```python
from build123d import *

# Parameters (mm, degrees)
SKETCH2_R          = 1.93
CUT_EXTRUDE1_DEPTH = 19.1
CIRPATTERN1_COUNT  = 16
SKETCH3_W          = 1.65
SKETCH3_H          = 14.001
CIRPATTERN2_COUNT  = 2
CIRPATTERN2_ANGLE  = 90


with BuildPart() as part:
    # Sketch1 → Revolve1 (revolve)
    with BuildSketch(Plane.XY):
        Polygon((-11.25, 6.35), (16.75, 6.35), (16.75, 14), (9.55, 14), (9.55, 11.66), (-9.55, 11.66), (-9.55, 10), (-11.25, 10), align=None)
    revolve(axis=Axis((0, 0, 0), (1, 0, 0)))

    # Sketch2 → Cut-Extrude1 (cut)
    with BuildSketch(Plane.ZY.offset(9.55)):
        with Locations((0, 11.93)):
            Circle(SKETCH2_R)
    cut_extrude1 = extrude(amount=-CUT_EXTRUDE1_DEPTH, mode=Mode.SUBTRACT)

    # CirPattern1: Cut-Extrude1 ×16 about axis
    cirpattern1_axis = Axis((0, 0, 0), (1, 0, 0))
    for i in range(1, CIRPATTERN1_COUNT):
        add(cut_extrude1.rotate(cirpattern1_axis, i * 360 / CIRPATTERN1_COUNT), mode=Mode.SUBTRACT)

    # Sketch3 → M4x0.7 Tapped Hole1 (revolve, cut)
    with BuildSketch(Plane(origin=(13.15, 0, 0), x_dir=(0, 0, -1), z_dir=(1, 0, 0))):
        with Locations((0.825, 7.0005)):
            Rectangle(SKETCH3_W, SKETCH3_H)
    m4x0_7_tapped_hole1 = revolve(axis=Axis((13.15, -6.35, 0), (0, 1, 0)), mode=Mode.SUBTRACT)

    # CirPattern2: M4x0.7 Tapped Hole1 ×2 about axis
    cirpattern2_axis = Axis((0, 0, 0), (-1, 0, 0))
    for i in range(1, CIRPATTERN2_COUNT):
        add(m4x0_7_tapped_hole1.rotate(cirpattern2_axis, i * CIRPATTERN2_ANGLE / (CIRPATTERN2_COUNT - 1)), mode=Mode.SUBTRACT)


solid = part.part
```
Geometry check sheet. Reference: the model listing, model coordinates, mm. A direction names the side the tool comes from. Round coordinates to 2 decimals unless told otherwise and drop trailing zeros. Order: outer loops, then holes, each group sorted by start corner. A loop starts at its lowest first (then second) coordinate and runs counter-clockwise, first axis right, second up. Notation, with made-up numbers: (5.5, -14.5) - (10.5, -14.5) arc R24 cw to (10.5, 7.5) - close; hole circle Ø6 at (54, 26.5). An arc over 180 degrees is marked (long way). Use a Markdown table: item, result. Add a question column.
1) Section check B-B (y = -4.5). Record the cut outline in (x, z).
2) Section check D-D (z = 8.5). Record the cut outline in (x, y).
3) Mould release check, pull along Z, two halves, no side actions. Record for faces 4 (the cylindrical face through (-0.134, 9.225, -3.861)), 5 (the cylindrical face through (-10.41, -2.17, -9.76)), 6 (the cylindrical face through (0, 0, 10)), 7 (the flat face through (-9.55, 6, -9)): released by +Z, released by -Z, zero draft, split by the parting line, or undercut.
4) Set-up check for faces 1 (the cylindrical face through (0, -10, 0)), 2 (the cylindrical face through (-0.134, 7.097, 7.046)), 3 (the flat face through (-9.55, -2, -10)): record each of +Z, -Z, +X, -X, +Y, -Y from which the full face is reachable in a straight line by a thin tool's end or side.
5) Thickness scan on line 1 along X through (y, z) = (10.75, 0); line 2 along X through (y, z) = (9.5, 0); line 3 along X through (y, z) = (-3, 12.25). Record the ranges inside material, lowest first.
6) Gauge pin test, flat ends, axial feed: P1, Ø1.8, axis at y = 10.5, z = -1, coming from the -X side; P2, Ø6, axis at x = 1, z = -1.5, coming from the +Y side; P3, Ø1.5, axis at x = -7, y = -11, coming from the -Z side; P4, Ø3, axis at x = 13.15, y = 0, coming from the -Z side. Record the tip position at first contact, or that the pin passes through.
7) Section check C-C (x = 13.15). Record the cut outline in (y, z), then the cut area to 3 significant figures.
Established:
| question | item | result |
|---|---|---|
| 1 | outline | (-11.25, -8.93) - (-9.55, -8.93) - (-9.55, -9.09) - (9.55, -9.09) - (9.55, -13.26) - (16.75, -13.26) - (16.75, -4.48) - (-11.25, -4.48) - close; (-11.25, 4.48) - (16.75, 4.48) - (16.75, 13.26) - (9.55, 13.26) - (9.55, 9.09) - (-9.55, 9.09) - (-9.55, 8.93) - (-11.25, 8.93) - close |
| 2 | outline | (-11.25, -5.27) - (-9.55, -5.27) - (-9.55, -6.51) - (9.55, -6.51) - (9.55, -11.12) - (16.75, -11.12) - (16.75, 11.12) - (9.55, 11.12) - (9.55, 6.51) - (-9.55, 6.51) - (-9.55, 5.27) - (-11.25, 5.27) - close |
| 3 | face 4 | undercut |
| 3 | face 5 | split by the parting line |
| 3 | face 6 | released by +Z |
| 3 | face 7 | zero draft |
| 4 | face 1 | -X, -Y |
| 4 | face 2 | -X |
| 4 | face 3 | -Z, -X, -Y |
| 5 | line 1 | 9.55 to 11.5, 14.8 to 16.75 |
| 5 | line 2 | -11.25 to 11.5, 14.8 to 16.75 |
| 5 | line 3 | 9.55 to 16.75 |
| 6 | P1 | x = -11.25 |
| 6 | P2 | y = 11.51 |
| 6 | P3 | z = -2.8 |
| 6 | P4 | z = 6.17 |
| 7 | outline | (-1.65, -13.9) - (-1.65, -6.13) arc R6.35 cw (long way) to (6.13, 1.65) - (13.9, 1.65) arc R14 ccw (long way) to start; (1.65, -13.9) arc R14 ccw to (13.9, -1.65) - (6.13, -1.65) arc R6.35 cw to (1.65, -6.13) - close |
| 7 | area | 438 mm2 |
